Here's how the part is built. I have some questions about the finished solid (model axes, mm). Round coordinates to 2 decimals unless told otherwise and drop trailing zeros. Write each loop counter-clockwise with the first axis right and the second up, starting at its lowest first coordinate (ties: lowest second). Pieces come first, ordered by that corner, then holes. Notation, with made-up numbers: (-37.75, -7) -> (-17.75, -7) arc R20 cw to (-17.75, 31) -> close; hole circle Ø1 at (-9.75, 49.25). An arc over 180 degrees is marked (long way). Answer as CSV lines item,"result".
from build123d import *

# Parameters (mm, degrees)
ESBO_O1_W                = 20
ESBO_O1_H                = 15
ESBO_O1_R                = 1.45
ESBO_O1_R_2              = 0.55
RESSALTO_EXTRUS_O1_DEPTH = 1.6
ESBO_O2_R                = 0.95
ESBO_O2_R_2              = 0.55
RESSALTO_EXTRUS_O2_DEPTH = 0.035
ESBO_O3_R                = 0.95
ESBO_O3_R_2              = 0.55
RESSALTO_EXTRUS_O3_DEPTH = 0.035


with BuildPart() as part:
    # Esboço1 → Ressalto-extrusão1 (new body)
    with BuildSketch(Plane(origin=(0, 0, 0), x_dir=(1, 0, 0), z_dir=(0, 1, 0))):
        Rectangle(ESBO_O1_W, ESBO_O1_H)
        with Locations((-7.5, 5)):
            Circle(ESBO_O1_R, mode=Mode.SUBTRACT)
        with Locations((7.5, 5)):
            Circle(ESBO_O1_R, mode=Mode.SUBTRACT)
        with Locations((-1.27, -6.5)):
            Circle(ESBO_O1_R_2, mode=Mode.SUBTRACT)
        with Locations((-3.81, -6.5)):
            Circle(ESBO_O1_R_2, mode=Mode.SUBTRACT)
        with Locations((-6.35, -6.5)):
            Circle(ESBO_O1_R_2, mode=Mode.SUBTRACT)
        with Locations((-8.89, -6.5)):
            Circle(ESBO_O1_R_2, mode=Mode.SUBTRACT)
        with Locations((1.27, -6.5)):
            Circle(ESBO_O1_R_2, mode=Mode.SUBTRACT)
        with Locations((3.81, -6.5)):
            Circle(ESBO_O1_R_2, mode=Mode.SUBTRACT)
        with Locations((6.35, -6.5)):
            Circle(ESBO_O1_R_2, mode=Mode.SUBTRACT)
        with Locations((8.89, -6.5)):
            Circle(ESBO_O1_R_2, mode=Mode.SUBTRACT)
    extrude(amount=RESSALTO_EXTRUS_O1_DEPTH)

    # Esboço2 → Ressalto-extrusão2 (add)
    with BuildSketch(Plane(origin=(0, 1.6, 0), x_dir=(1, 0, 0), z_dir=(0, 1, 0))):
        with Locations((-6.35, -6.5)):
            Circle(ESBO_O2_R)
        with Locations((-6.35, -6.5)):
            Circle(ESBO_O2_R_2, mode=Mode.SUBTRACT)
        with Locations((-8.89, -6.5)):
            Circle(ESBO_O2_R)
        with Locations((-8.89, -6.5)):
            Circle(ESBO_O2_R_2, mode=Mode.SUBTRACT)
        with Locations((-3.81, -6.5)):
            Circle(ESBO_O2_R)
        with Locations((-3.81, -6.5)):
            Circle(ESBO_O2_R_2, mode=Mode.SUBTRACT)
        with Locations((-1.27, -6.5)):
            Circle(ESBO_O2_R)
        with Locations((-1.27, -6.5)):
            Circle(ESBO_O2_R_2, mode=Mode.SUBTRACT)
        with Locations((1.27, -6.5)):
            Circle(ESBO_O2_R)
        with Locations((1.27, -6.5)):
            Circle(ESBO_O2_R_2, mode=Mode.SUBTRACT)
        with Locations((3.81, -6.5)):
            Circle(ESBO_O2_R)
        with Locations((3.81, -6.5)):
            Circle(ESBO_O2_R_2, mode=Mode.SUBTRACT)
        with Locations((6.35, -6.5)):
            Circle(ESBO_O2_R)
        with Locations((6.35, -6.5)):
            Circle(ESBO_O2_R_2, mode=Mode.SUBTRACT)
        with Locations((8.89, -6.5)):
            Circle(ESBO_O2_R)
        with Locations((8.89, -6.5)):
            Circle(ESBO_O2_R_2, mode=Mode.SUBTRACT)
    extrude(amount=RESSALTO_EXTRUS_O2_DEPTH)

    # Esboço3 → Ressalto-extrusão3 (add)
    with BuildSketch(Plane.XZ):
        with Locations((8.89, 6.5)):
            Circle(ESBO_O3_R)
        with Locations((8.89, 6.5)):
            Circle(ESBO_O3_R_2, mode=Mode.SUBTRACT)
        with Locations((6.35, 6.5)):
            Circle(ESBO_O3_R)
        with Locations((6.35, 6.5)):
            Circle(ESBO_O3_R_2, mode=Mode.SUBTRACT)
        with Locations((3.81, 6.5)):
            Circle(ESBO_O3_R)
        with Locations((3.81, 6.5)):
            Circle(ESBO_O3_R_2, mode=Mode.SUBTRACT)
        with Locations((1.27, 6.5)):
            Circle(ESBO_O3_R)
        with Locations((1.27, 6.5)):
            Circle(ESBO_O3_R_2, mode=Mode.SUBTRACT)
        with Locations((-1.27, 6.5)):
            Circle(ESBO_O3_R)
        with Locations((-1.27, 6.5)):
            Circle(ESBO_O3_R_2, mode=Mode.SUBTRACT)
        with Locations((-3.81, 6.5)):
            Circle(ESBO_O3_R)
        with Locations((-3.81, 6.5)):
            Circle(ESBO_O3_R_2, mode=Mode.SUBTRACT)
        with Locations((-6.35, 6.5)):
            Circle(ESBO_O3_R)
        with Locations((-6.35, 6.5)):
            Circle(ESBO_O3_R_2, mode=Mode.SUBTRACT)
        with Locations((-8.89, 6.5)):
            Circle(ESBO_O3_R)
        with Locations((-8.89, 6.5)):
            Circle(ESBO_O3_R_2, mode=Mode.SUBTRACT)
    extrude(amount=RESSALTO_EXTRUS_O3_DEPTH)


solid = part.part
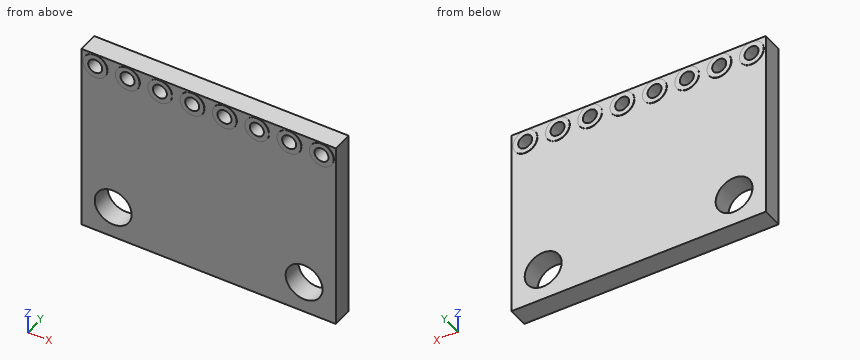
Item 1: Suppose I cut it at B-B, the plane y = 1.35. State how many separate pieces and enclosed holes the cut face has, then the cut area to 3 significant figures.
Results found:
separate pieces,"1"
enclosed holes,"10"
area,"279 mm²"
Item 2: Suppose I cut it at A-A, the plane x = -1.27. List the corners of the cut face in (y, z) for me (3 decimals), then the cut area to 3 significant figures.
Results found:
outline,"(-0.035, 5.55) -> (0, 5.55) -> (0, -7.5) -> (1.6, -7.5) -> (1.6, 5.55) -> (1.635, 5.55) -> (1.635, 5.95) -> (-0.035, 5.95) -> close; (-0.035, 7.05) -> (1.635, 7.05) -> (1.635, 7.45) -> (1.6, 7.45) -> (1.6, 7.5) -> (0, 7.5) -> (0, 7.45) -> (-0.035, 7.45) -> close"
area,"22.3 mm²"
Item 3: I need wall thicknesses on L1, parallel to Z at x = 6.35, y = 1.2; L2, parallel to Z at x = -8.5, y = 0.8; L3, parallel to X at y = 1.4, z = -5.5. Which ranges of each line are inside material? Lowest first, please.
Results found:
L1,"z = -7.5 to -5.88, -4.12 to 5.95, 7.05 to 7.5"
L2,"z = -7.5 to -6.05, -3.95 to 6.11, 6.89 to 7.5"
L3,"x = -10 to -8.86, -6.14 to 6.14, 8.86 to 10"
Item 4: Will these pins go through, and if not, where does the flat tip stop? pin 1 (0.7 mm diameter, centred on x = -8.89, z = 6.5, fed in from -Y); pin 2 (4 mm diameter, centred on x = 3, z = -5.5, fed in from -Y).
Results found:
pin 1,"passes through"
pin 2,"stops at y = 0"
Item 5: Suppose I cut it at C-C, the plane z = -5.5. List the corners of the cut face in (x, y) for me, then the cut area to 3 significant figures.
Results found:
outline,"(-10, 0) -> (-8.86, 0) -> (-8.86, 1.6) -> (-10, 1.6) -> close; (-6.14, 0) -> (6.14, 0) -> (6.14, 1.6) -> (-6.14, 1.6) -> close; (8.86, 0) -> (10, 0) -> (10, 1.6) -> (8.86, 1.6) -> close"
area,"23.3 mm²"
Item 6: Suppose I cut it at D-D, the plane x = -6.5. List the corners of the cut face in (y, z) for me (3 decimals), then the cut area to 3 significant figures.
Results found:
outline,"(-0.035, 5.562) -> (0, 5.562) -> (0, -3.95) -> (1.6, -3.95) -> (1.6, 5.562) -> (1.635, 5.562) -> (1.635, 5.971) -> (-0.035, 5.971) -> close; (-0.035, 7.029) -> (1.635, 7.029) -> (1.635, 7.438) -> (1.6, 7.438) -> (1.6, 7.5) -> (0, 7.5) -> (0, 7.438) -> (-0.035, 7.438) -> close; (0, -7.5) -> (1.6, -7.5) -> (1.6, -6.05) -> (0, -6.05) -> close"
area,"19.0 mm²"
